Source: CAD feature listing. Evaluate the final solid. Frame: model axes, mm. A direction names the side the tool comes from. Give positions to 0.01 mm unless a question says otherwise; leave off trailing zeros. Write each loop counter-clockwise with the first axis right and the second up, starting at its lowest first coordinate (ties: lowest second). Pieces come first, ordered by that corner, then holes. Notation, with made-up numbers: (-25.75, 73) - (-14.75, 73) arc R23 cw to (-14.75, 95) - close; hole circle Ø11 at (81.25, 32). An arc over 180 degrees is marked (long way). One line per question, with ' | ' between items. Start each with the question number.
(1) Draft query along Y for faces 3 (the cylindrical face through (-2.868, -259.836, -4.498)), 4 (the cylindrical face through (4.16, -23.08, 4.51)). Return one class per face: +Y half, -Y half, draft (parallel to the pull), parting line (faces both ways), or undercut.
(2) Pin query (flat end, axial travel): pin 1 (3 mm diameter, centred on x = 2, y = -429, fed in from +Z); pin 2 (2 mm diameter, centred on y = -183, z = -4, fed in from -X); pin 3 (3 mm diameter, centred on x = -4, y = -359.5, fed in from +Z); pin 4 (6.5 mm diameter, centred on x = 0, z = 0, fed in from +Y). Return the tip coordinate at first contact, or that it passes through.
(3) Access query for faces 1 (the cylindrical face through (0.8, -259.8, -6.3)), 2 (the cylindrical face through (4.16, -505.68, 4.51)). Directions: +Z, -Z, +X, -X, +Y, -Y. A direction counts if a zero-diameter tool reaches every point of the face in a straight line with its end or side. Return the directions, or none.
(4) Section A-A, the plane z = 0. Return loops of the section in (x, y), plus the area to 3 significant figures.
(5) Section C-C, the plane y = -237.5. Return loops of the section in (x, z), plus the area to 3 significant figures.
(6) Ray query, line 1 (X direction, y = -269, z = 0); line 2 (Y direction, x = -3.5, z = 5.25). Return the intervals inside material, ascending. Write a range as [from, to].
(7) Section B-B, the plane x = 0. Return loops of the section in (y, z).
(8) Section D-D, the plane y = -25.4. Return loops of the section in (x, z).
```python
from build123d import *

# Parameters (mm, degrees)
SKETCH1_W                             = 1.016
SKETCH1_H                             = 527.05
F_3_8_0_375_DIAMETER_HOLE1_AT_2_COUNT = 2
F_3_8_0_375_DIAMETER_HOLE1_AT_2_PITCH = 482.6


with BuildPart() as part:
    # Sketch1 → Revolve1 (revolve)
    with BuildSketch(Plane.XY):
        with Locations((-5.842, -263.525)):
            Rectangle(SKETCH1_W, SKETCH1_H)
    revolve(axis=Axis((0, 0, 0), (0, -1, 0)))

    # Sketch3 → 3/8 (0.375) Diameter Hole1 (revolve, cut)
    with BuildSketch(Plane(origin=(0, -508, 0), x_dir=(0, 1, 0), z_dir=(1, 0, 0))):
        Polygon((0, 0), (0, 9.211598698), (4.7625, 6.35), (4.7625, 0), align=None)
    f_3_8_0_375_diameter_hole1 = revolve(axis=Axis((0, -508, -6.35), (0, 0, 1)), mode=Mode.SUBTRACT)

    # 3/8 (0.375) Diameter Hole1 at 2: 3/8 (0.375) Diameter Hole1 ×2
    with Locations(*[(0, i * F_3_8_0_375_DIAMETER_HOLE1_AT_2_PITCH, 0) for i in range(1, F_3_8_0_375_DIAMETER_HOLE1_AT_2_COUNT)]):
        add(f_3_8_0_375_diameter_hole1, mode=Mode.SUBTRACT)


solid = part.part
```
Check sheet entries:
1) face 3: draft | face 4: undercut
2) pin 1: z = 6.33 | pin 2: x = -5.6 | pin 3: z = 5.84 | pin 4: through
3) face 1: +Y, -Y | face 2: +Z
4) outline: (-6.35, -527.05) - (-5.33, -527.05) - (-5.33, 0) - (-6.35, 0) - close; (5.33, -527.05) - (6.35, -527.05) - (6.35, 0) - (5.33, 0) - close | area: 1,070 mm²
5) outline: circle Ø12.7 at (0, 0); hole circle Ø10.67 at (0, 0) | area: 37.3 mm²
6) line 1: [-6.35, -5.33], [5.33, 6.35] | line 2: [-527.05, -511.23], [-504.77, -28.63], [-22.17, 0]
7) outline: (-527.05, -6.35) - (0, -6.35) - (0, -5.33) - (-527.05, -5.33) - close; (-527.05, 5.33) - (-512.76, 5.33) - (-512.76, 6.35) - (-527.05, 6.35) - close; (-503.24, 5.33) - (-30.16, 5.33) - (-30.16, 6.35) - (-503.24, 6.35) - close; (-20.64, 5.33) - (0, 5.33) - (0, 6.35) - (-20.64, 6.35) - close
8) outline: (-4.76, 2.4) - (-4.76, 4.2) arc R6.35 ccw (long way) to (4.76, 4.2) - (4.76, 2.4) arc R5.33 cw (long way) to start
